from build123d import *

# Parameters (mm, degrees)
ESQUISSE1_W             = 140
ESQUISSE1_H             = 140
BOSS_EXTRU_1_DEPTH      = 20
ESQUISSE2_W             = 120
ESQUISSE2_H             = 120
ENL_V_MAT_EXTRU_1_DEPTH = 10
CONG_1_R                = 10
CONG_2_R                = 10
ESQUISSE3_R             = 6.5
BOSS_EXTRU_2_DEPTH      = 10
CONG_3_R                = 1


with BuildPart() as part:
    # Esquisse1 → Boss.-Extru.1 (new body)
    with BuildSketch(Plane.XY):
        Rectangle(ESQUISSE1_W, ESQUISSE1_H)
    extrude(amount=BOSS_EXTRU_1_DEPTH)

    # Esquisse2 → Enlèv. mat.-Extru.1 (cut)
    with BuildSketch(Plane.XY.offset(20)):
        Rectangle(ESQUISSE2_W, ESQUISSE2_H)
    extrude(amount=-ENL_V_MAT_EXTRU_1_DEPTH, mode=Mode.SUBTRACT)

    # Congé1
    cong_1_edges = [part.edges().sort_by_distance(p)[0] for p in [
        (60, 60, 15),
        (60, -60, 15),
        (-60, -60, 15),
        (-60, 60, 15),
    ]]
    fillet(cong_1_edges, radius=CONG_1_R)

    # Congé2
    cong_2_edges = [part.edges().sort_by_distance(p)[0] for p in [
        (70, -70, 10),
        (-70, -70, 10),
        (-70, 70, 10),
        (70, 70, 10),
    ]]
    fillet(cong_2_edges, radius=CONG_2_R)

    # Esquisse3 → Boss.-Extru.2 (add)
    with BuildSketch(Plane.XY.offset(10)):
        with Locations(Location((0, 0, 0), (0, 0, 180))):
            Circle(ESQUISSE3_R)
    extrude(amount=BOSS_EXTRU_2_DEPTH)

    # Congé3
    cong_3_edges = [part.edges().sort_by_distance(p)[0] for p in [
        (6.5, 0, 20),
    ]]
    fillet(cong_3_edges, radius=CONG_3_R)


solid = part.part
Part model, mm, in its own coordinate system. A direction names the side the tool comes from. Coordinates: 2 decimals unless noted, no trailing zeros. Order: outer loops, then holes, each group sorted by start corner. A loop starts at its lowest first (then second) coordinate and runs counter-clockwise, first axis right, second up. Notation, with made-up numbers: M 4.5,70 L 22.5,70 A25 ccw 22.5,92 Z; hole C 79,80.5 d9. An arc over 180 degrees is marked long. Use a Markdown table: item, result.
(1) Tool access for faces 1 (the cylindrical face through (56.99, -57.15, 14.93)), 2 (the cylindrical face through (66.99, -67.15, 10.14)): list every direction of +Z, -Z, +X, -X, +Y, -Y with a clear straight run to the whole face (end or side of a thin tool).
A:
| item | result |
|---|---|
| face 1 | +Z |
| face 2 | +Z, -Z, +X, -Y |
(2) Cut at A-A on z = 15.5. Write the cut outline in (x, y), then the cut area to 3 significant figures.
A:
| item | result |
|---|---|
| outline | M -70,-60 A10 ccw -60,-70 L 60,-70 A10 ccw 70,-60 L 70,60 A10 ccw 60,70 L -60,70 A10 ccw -70,60 Z; C 0,0 d13; hole M -60,-50 A10 ccw -50,-60 L 50,-60 A10 ccw 60,-50 L 60,50 A10 ccw 50,60 L -50,60 A10 ccw -60,50 Z |
| area | 5,330 mm^2 |
(3) Pull direction X, two halves, no side cores. Call faces 3 (the cylindrical face through (-67.15, 66.99, 10.14)), 4 (the flat face through (-1, -60, 15)), 5 (the flat face through (-1, 70, 10)): released by +X, released by -X, zero draft, split by the parting line, or undercut.
A:
| item | result |
|---|---|
| face 3 | released by -X |
| face 4 | undercut |
| face 5 | zero draft |
(4) Flat gauge pin, fed straight in: pin 1 (6 mm diameter, centred on x = -35, y = -23.5, fed in from +Z). Where does the tip first touch, or does it go through?
A:
| item | result |
|---|---|
| pin 1 | stops at z = 10 |
(5) Probe L1, parallel to X at y = 9, z = 15.75; L2, parallel to X at y = 2.5, z = 15. List the from-to ranges inside material, lowest first.
A:
| item | result |
|---|---|
| L1 | x = -70 to -60, 60 to 70 |
| L2 | x = -70 to -60, -6 to 6, 60 to 70 |
(6) Cut at D-D on x = 0. Write the cut outline in (y, z).
A:
| item | result |
|---|---|
| outline | M -70,0 L 70,0 L 70,20 L 60,20 L 60,10 L 6.5,10 L 6.5,19 A1 ccw 5.5,20 L -5.5,20 A1 ccw -6.5,19 L -6.5,10 L -60,10 L -60,20 L -70,20 Z |
(7) Cut at B-B on x = -44. Write the cut outline in (y, z).
A:
| item | result |
|---|---|
| outline | M -70,0 L 70,0 L 70,20 L 60,20 L 60,10 L -60,10 L -60,20 L -70,20 Z |
